from build123d import *

# Parameters (mm, degrees)
F0_W     = 23
F0_H     = 23
F1_DEPTH = 1
F2_DEPTH = 11.8
F3_W     = 2.7
F3_H     = 11.8
F4_DEPTH = 32.401


with BuildPart() as f1:
    # F0 (on Top) → F1 (new body)
    with BuildSketch(Plane.XY):
        with Locations((3.442476, 0.669988)):
            Rectangle(F0_W, F0_H)
        Polygon((14.942476, -10.830012), (-8.057524, -10.830012), (-12.757524, -10.830012), (-12.757524, -15.530012), (14.942476, -15.530012), align=None)
        Polygon((-8.057524, -10.830012), (-8.057524, 12.169988), (-8.057524, 16.869988), (-12.757524, 16.869988), (-12.757524, -10.830012), align=None)
        Polygon((-8.057524, 16.869988), (-8.057524, 12.169988), (14.942476, 12.169988), (19.642476, 12.169988), (19.642476, 16.869988), align=None)
        Polygon((19.642476, 12.169988), (14.942476, 12.169988), (14.942476, -10.830012), (14.942476, -15.530012), (19.642476, -15.530012), align=None)
    extrude(amount=-F1_DEPTH)

    # F0 (on Top) → F2 (join)
    with BuildSketch(Plane.XY):
        Polygon((-8.057524, 16.869988), (-8.057524, 12.169988), (14.942476, 12.169988), (19.642476, 12.169988), (19.642476, 16.869988), align=None)
        Polygon((-8.057524, -10.830012), (-8.057524, 12.169988), (-8.057524, 16.869988), (-12.757524, 16.869988), (-12.757524, -10.830012), align=None)
        Polygon((19.642476, 12.169988), (14.942476, 12.169988), (14.942476, -10.830012), (14.942476, -15.530012), (19.642476, -15.530012), align=None)
        Polygon((14.942476, -10.830012), (-8.057524, -10.830012), (-12.757524, -10.830012), (-12.757524, -15.530012), (14.942476, -15.530012), align=None)
    extrude(amount=F2_DEPTH)

    # F3 (on face) → F4 (cut, through all)
    with BuildSketch(Plane.XZ.offset(15.530012)):
        with Locations((-2.307524, 5.9)):
            Rectangle(F3_W, F3_H)
    extrude(amount=-F4_DEPTH, mode=Mode.SUBTRACT)


solid = f1.part
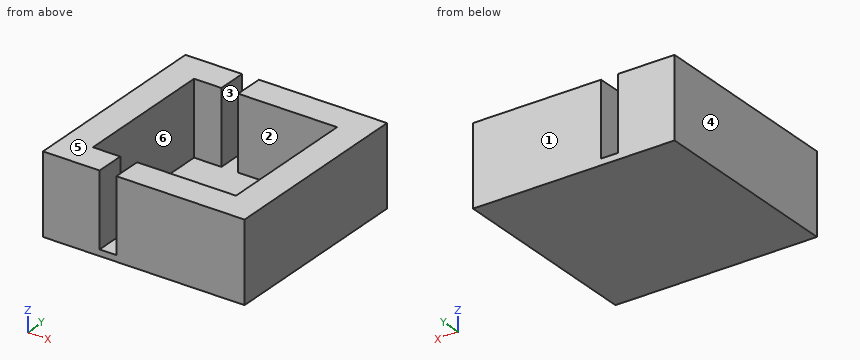
Geometry: final body of the model. Coordinates: model frame, mm. Face numbers are marked on the shaded views. A direction names the side the tool comes from. Coordinates: 2 decimals unless noted, no trailing zeros. Loops run counter-clockwise (first coordinate to the right, second up) from the corner with the lowest first, then second, coordinate; pieces in that order, holes last. Notation, with made-up numbers: (54.25, 28.5) - (59.25, 28.5) arc R23 cw to (59.25, 51.5) - close; hole circle Ø11 at (-40, 55). An arc over 180 degrees is marked (long way). Put each result on its own line as item: value. Start each with the question number.
Q1. Line query: line 1 (Y direction, x = 3.5, z = 3.5); line 2 (X direction, y = 8.5, z = 1); line 3 (X direction, y = -12, z = 4). Output: solid intervals per line, ascending.
Q2. Cut plane B-B, the plane y = -3. Return loops of the section in (x, z).
Q3. Cut plane C-C, the plane x = 7.5. Return loops of the section in (y, z).
Q4. Set-up query: the marked faces 1, 2 and 3. Return all of +Z, -Z, +X, -X, +Y, -Y with unobstructed straight access to the full face (end or side cutting, diameter ignored); none if empty.
Q5. Pull-direction query (X, two-part tool) for the marked faces 4, 5 and 6; classes: released by +X, released by -X, zero draft, split by the parting line, or undercut.
Q6. Cut plane A-A, the plane z = 3. Return loops of the section in (x, y), and give its area (3 significant figures).
Q7. Pin query (flat end, axial travel): pin 1 Ø10 at (x, y) = (-3, -5.5) entering from +Z; pin 2 Ø18.5 at (x, y) = (-1, 5) entering from +Z. Return the tip coordinate at first contact, or that it passes through.
Filled sheet:
1. line 1: -15.53 to -10.83, 12.17 to 16.87
1. line 2: -12.76 to -8.06, 14.94 to 19.64
1. line 3: -12.76 to -3.66, -0.96 to 19.64
2. outline: (-12.76, -1) - (19.64, -1) - (19.64, 11.8) - (14.94, 11.8) - (14.94, 0) - (-8.06, 0) - (-8.06, 11.8) - (-12.76, 11.8) - close
3. outline: (-15.53, -1) - (16.87, -1) - (16.87, 11.8) - (12.17, 11.8) - (12.17, 0) - (-10.83, 0) - (-10.83, 11.8) - (-15.53, 11.8) - close
4. face 1: +Z, -Z, +X, -X, +Y
4. face 2: +Z
4. face 3: +Z, +Y, -Y
5. face 4: released by -X
5. face 5: zero draft
5. face 6: undercut
6. outline: (-12.76, -15.53) - (-3.66, -15.53) - (-3.66, -10.83) - (-8.06, -10.83) - (-8.06, 12.17) - (-3.66, 12.17) - (-3.66, 16.87) - (-12.76, 16.87) - close; (-0.96, -15.53) - (19.64, -15.53) - (19.64, 16.87) - (-0.96, 16.87) - (-0.96, 12.17) - (14.94, 12.17) - (14.94, -10.83) - (-0.96, -10.83) - close
6. area: 495 mm²
7. pin 1: z = 0
7. pin 2: z = 11.8
